Check sheet for the modelled part. Datum: model origin and axes. Units: mm. Face numbers are marked on the shaded views. A direction names the side the tool comes from. Give positions to 0.01 mm unless a question says otherwise; leave off trailing zeros. Write each loop counter-clockwise with the first axis right and the second up, starting at its lowest first coordinate (ties: lowest second). Pieces come first, ordered by that corner, then holes. Notation, with made-up numbers: (33.5, 14) -> (66.5, 14) arc R20 ccw to (66.5, 28) -> close; hole circle Ø3 at (4.5, 23.25). An arc over 180 degrees is marked (long way). Return JSON: item names as keys, results as strings.
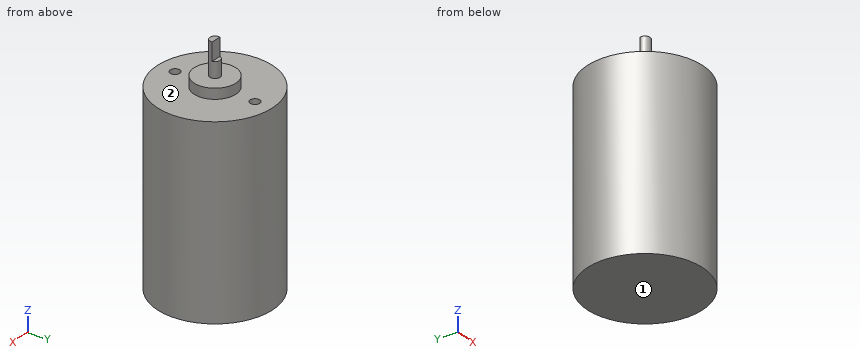
from build123d import *

# Parameters (mm, degrees)
SKETCH1_R           = 17.9
BOSS_EXTRUDE1_DEPTH = 57.5
SKETCH2_R           = 6.5
BOSS_EXTRUDE2_DEPTH = 3.175
SKETCH3_R           = 1.5875
BOSS_EXTRUDE3_DEPTH = 10.325
CUT_EXTRUDE1_DEPTH  = 5.5
SKETCH5_R           = 1.5
CUT_EXTRUDE2_DEPTH  = 5.5


with BuildPart() as part:
    # Sketch1 → Boss-Extrude1 (new body)
    with BuildSketch(Plane.XY):
        Circle(SKETCH1_R)
    extrude(amount=BOSS_EXTRUDE1_DEPTH)

    # Sketch2 → Boss-Extrude2 (add)
    with BuildSketch(Plane.XY.offset(57.5)):
        Circle(SKETCH2_R)
    extrude(amount=BOSS_EXTRUDE2_DEPTH)

    # Sketch3 → Boss-Extrude3 (add)
    with BuildSketch(Plane.XY.offset(60.675)):
        with Locations(Location((0, 0, 0), (0, 0, 180))):
            Circle(SKETCH3_R)
    extrude(amount=BOSS_EXTRUDE3_DEPTH)

    # Sketch4 → Cut-Extrude1 (cut)
    with BuildSketch(Plane.XY.offset(71)):
        with BuildLine():
            Line((-1.555064123, 0.319267636), (1.555064123, 0.319267636))
            ThreePointArc((1.555064123, 0.319267636), (0, 1.603005123), (-1.555064123, 0.319267636))
        make_face()
    extrude(amount=-CUT_EXTRUDE1_DEPTH, mode=Mode.SUBTRACT)

    # Sketch5 → Cut-Extrude2 (cut)
    with BuildSketch(Plane.XY.offset(57.5)):
        with Locations((0, 12.5)):
            Circle(SKETCH5_R)
        with Locations((0, -12.5)):
            Circle(SKETCH5_R)
    extrude(amount=-CUT_EXTRUDE2_DEPTH, mode=Mode.SUBTRACT)


solid = part.part
(1) Set-up check for the marked faces 1 and 2: record each of +Z, -Z, +X, -X, +Y, -Y from which the full face is reachable in a straight line by a thin tool's end or side.
Reply:
{"face 1": "-Z, +X, -X, +Y, -Y", "face 2": "+Z"}
(2) Cross-section at B-B on y = -4. Enter the section's corners in (x, z) (3 decimals), then the cut area to 3 significant figures.
Reply:
{"outline": "(-17.447, 0) -> (17.447, 0) -> (17.447, 57.5) -> (5.123, 57.5) -> (5.123, 60.675) -> (-5.123, 60.675) -> (-5.123, 57.5) -> (-17.447, 57.5) -> close", "area": "2,040 mm^2"}
(3) Thickness scan on L1, parallel to Y at x = 0, z = 54.75; L2, parallel to Z at x = -12.5, y = -12.5; L3, parallel to Z at x = -1, y = -3.5 (3 decimals). Record the ranges inside material, lowest first.
Reply:
{"L1": "-17.9 to -14, -11 to 11, 14 to 17.9", "L2": "0 to 57.5", "L3": "0 to 60.675"}
(4) Cross-section at A-A on x = 0. Enter the section's corners in (y, z) (1 decimal).
Reply:
{"outline": "(-17.9, 0) -> (17.9, 0) -> (17.9, 57.5) -> (14, 57.5) -> (14, 52) -> (11, 52) -> (11, 57.5) -> (6.5, 57.5) -> (6.5, 60.7) -> (1.6, 60.7) -> (1.6, 65.5) -> (0.3, 65.5) -> (0.3, 71) -> (-1.6, 71) -> (-1.6, 60.7) -> (-6.5, 60.7) -> (-6.5, 57.5) -> (-11, 57.5) -> (-11, 52) -> (-14, 52) -> (-14, 57.5) -> (-17.9, 57.5) -> close"}
(5) Cross-section at C-C on z = 59. Enter the section's corners in (x, y).
Reply:
{"outline": "circle Ø13 at (0, 0)"}
(6) Cross-section at D-D on x = -5. Enter the section's corners in (y, z) (1 decimal), then the cut area to 3 significant figures.
Reply:
{"outline": "(-17.2, 0) -> (17.2, 0) -> (17.2, 57.5) -> (4.2, 57.5) -> (4.2, 60.7) -> (-4.2, 60.7) -> (-4.2, 57.5) -> (-17.2, 57.5) -> close", "area": "2,000 mm^2"}
(7) Depth check by flat-ended pin: pin 1 Ø1.5 at (x, z) = (8, 18.5) entering from -Y; pin 2 Ø0.9 at (x, z) = (0.5, 68) entering from +Y; pin 3 Ø0.9 at (x, y) = (-0.5, 12) entering from +Z. Enter the tip coordinate at first touch or a pass-through.
Reply:
{"pin 1": "y = -16.37", "pin 2": "y = 0.32", "pin 3": "z = 52"}
